CAD build for the part. Positions are in the model's coordinates, mm. Face numbers are marked on the shaded views. Coordinates: 2 decimals unless noted, no trailing zeros. Write each loop counter-clockwise with the first axis right and the second up, starting at its lowest first coordinate (ties: lowest second). Pieces come first, ordered by that corner, then holes. Notation, with made-up numbers: M 82,-29.75 L 103,-29.75 A13 ccw 103,-4.75 Z; hole C -6,41 d8. An arc over 180 degrees is marked long. Put each result on its own line as item: value. Start each with the question number.
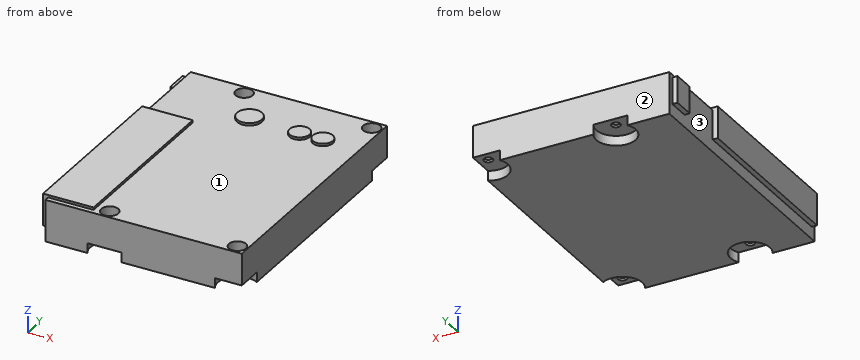
```python
from build123d import *

# Parameters (mm, degrees)
F0_W      = 80
F0_H      = 106
F0_R      = 1.8
F1_DEPTH  = 1
F2_W      = 20.6
F2_H      = 72.4
F3_DEPTH  = 13
F4_W      = 10
F4_H      = 8.9
F5_DEPTH  = 10.9
F6_R      = 5.1
F6_R_2    = 4.1
F7_DEPTH  = 13
F9_DEPTH  = 4
F10_W     = 80
F10_H     = 106
F10_R     = 3.5
F11_DEPTH = 12


with BuildPart() as f1:
    # F0 (on Top) → F1 (new body)
    with BuildSketch(Plane.XY):
        Rectangle(F0_W, F0_H)
        with Locations((-16, -49)):
            Circle(F0_R, mode=Mode.SUBTRACT)
        with Locations((36, -49)):
            Circle(F0_R, mode=Mode.SUBTRACT)
        with Locations((-16, 49)):
            Circle(F0_R, mode=Mode.SUBTRACT)
        with Locations((36, 49)):
            Circle(F0_R, mode=Mode.SUBTRACT)
    extrude(amount=-F1_DEPTH)

    # F2 (on face) → F3 (join)
    with BuildSketch(Plane.XY):
        with Locations((-31.8, -14.81)):
            Rectangle(F2_W, F2_H)
    extrude(amount=F3_DEPTH)

    # F4 (on face) → F5 (join)
    with BuildSketch(Plane.XY):
        with Locations((-37.1, 46.35)):
            Rectangle(F4_W, F4_H)
    extrude(amount=F5_DEPTH)

    # F6 (on face) → F7 (join)
    with BuildSketch(Plane.XY):
        with Locations((-5.3, 33.8)):
            Circle(F6_R)
        with Locations((15.8, 32.6)):
            Circle(F6_R_2)
        with Locations((25.24, 32.6)):
            Circle(F6_R_2)
    extrude(amount=F7_DEPTH)

    # F8 (on face) → F9 (join)
    with BuildSketch(Plane(origin=(0, 0, -1), x_dir=(1, 0, 0), z_dir=(0, 0, -1))):
        with BuildLine():
            Line((-22.928203, 53), (-40, 53))
            Line((-40, 53), (-40, -53))
            Line((-40, -53), (-22.928203, -53))
            ThreePointArc((-22.928203, -53), (-16, -41), (-9.071797, -53))
            Line((-9.071797, -53), (29.071797, -53))
            ThreePointArc((29.071797, -53), (30.343146, -43.343146), (40, -42.071797))
            Line((40, -42.071797), (40, 42.071797))
            ThreePointArc((40, 42.071797), (30.343146, 43.343146), (29.071797, 53))
            Line((29.071797, 53), (-9.071797, 53))
            ThreePointArc((-9.071797, 53), (-16, 41), (-22.928203, 53))
        make_face()
    extrude(amount=F9_DEPTH)

    # F10 (on face) → F11 (join)
    with BuildSketch(Plane.XY):
        Rectangle(F10_W, F10_H)
        with Locations((-16, -49)):
            Circle(F10_R, mode=Mode.SUBTRACT)
        with Locations((36, -49)):
            Circle(F10_R, mode=Mode.SUBTRACT)
        with Locations((-16, 49)):
            Circle(F10_R, mode=Mode.SUBTRACT)
        with Locations((36, 49)):
            Circle(F10_R, mode=Mode.SUBTRACT)
    extrude(amount=F11_DEPTH)


solid = f1.part
```
(1) Drill centre lines: line 1 (Y direction, x = 36, z = 4.75); line 2 (Y direction, x = 36, z = -0.8); line 3 (X direction, y = -48.5, z = -0.75). Where is each one in solid material? Low to high. Write a range as [from, to].
(2) Slice it at A-A, the plane z = 7. Write the cut outline in (x, y).
(3) Two-plate mould, pull along Y, no slides. Class the marked faces 1, 2 and 3: +Y half, -Y half, draft (parallel to the pull), parting line (faces both ways), or undercut.
(4) Drop flat-ended pins along their axis: pin 1 (10 mm diameter, centred on x = 0.5, y = -0.5, fed in from +Z); pin 2 (6.5 mm diameter, centred on x = 36, y = 49, fed in from +Z); pin 3 (11 mm diameter, centred on x = -16, y = 49, fed in from -Z). Give the stop position or say it passes through.
(5) Slice it at D-D, the plane x = 15.8. Write the cut outline in (y, z).
(6) Slice it at B-B, the plane y = 49. State how many separate pieces and enclosed holes the cut face has, then the cut area to 3 significant figures.
(7) Slice it at C-C, the plane y = -1.5. Write the cut outline in (x, z).
Result set:
1. line 1: y = [-53, -52.5], [-45.5, 45.5], [52.5, 53]
1. line 2: y = [-53, -50.8], [-47.2, 47.2], [50.8, 53]
1. line 3: x = [-40, -17.73], [-14.27, 34.27], [37.73, 40]
2. outline: M -42.1,-51.01 L -40,-51.01 L -40,-53 L 40,-53 L 40,53 L -40,53 L -40,50.8 L -42.1,50.8 L -42.1,41.9 L -40,41.9 L -40,21.39 L -42.1,21.39 Z; hole C -16,-49 d7; hole C -16,49 d7; hole C 36,-49 d7; hole C 36,49 d7
3. face 1: draft
3. face 2: +Y half
3. face 3: undercut
4. pin 1: stops at z = 12
4. pin 2: stops at z = 0
4. pin 3: stops at z = -1
5. outline: M -53,-5 L 53,-5 L 53,12 L 36.7,12 L 36.7,13 L 28.5,13 L 28.5,12 L -53,12 Z
6. separate pieces: 3
6. enclosed holes: 0
6. area: 1,100 mm^2
7. outline: M -42.1,0 L -40,0 L -40,-5 L 40,-5 L 40,12 L -21.5,12 L -21.5,13 L -42.1,13 Z
